Check sheet for the modelled part. Datum: model origin and axes. Units: mm. Face numbers are marked on the shaded views. Coordinates: 2 decimals unless noted, no trailing zeros. Loops run counter-clockwise (first coordinate to the right, second up) from the corner with the lowest first, then second, coordinate; pieces in that order, holes last. Notation, with made-up numbers: (75.25, 12) -> (90.25, 12) arc R20 cw to (90.25, 26) -> close; hole circle Ø4 at (-31, 27). An arc over 180 degrees is marked (long way). Use one line per item in the form item = value.
Autodesk Inventor part; units mm, degrees
ref_plane "YZ Plane" through (0, 0, 0) normal (1, 0, 0) x (0, 1, 0)
ref_plane "XZ Plane" through (0, 0, 0) normal (0, 1, 0) x (-1, 0, 0)
ref_plane "XY Plane" through (0, 0, 0) normal (0, 0, 1) x (1, 0, 0)
sketch "Boceto1" plane through (0, 0, 0) normal (0, 1, 0) x (-1, 0, 0)
  line L0 (-15, 25) -> (15, 25)
  line L1 (15, 25) -> (15, -25)
  line L2 (15, -25) -> (-15, -25)
  line L3 (-15, -25) -> (-15, 25)
  line L4 (-15, 25) -> (15, -25) construction
  line L5 (15, 25) -> (-15, -25) construction
  point P0 (0, 0)
  dimension "d0" = 50
  dimension "d1" = 30
extrude "Extrusión1" add sketch "Boceto1" along normal blind 8
fillet "Empalme1" radius 2 4 edges at (15, 4, 25) (-15, 4, 25) (15, 4, -25) (-15, 4, -25)
sketch "Boceto2" plane through (0, 8, 0) normal (0, 1, 0) x (1, 0, 0)
  circle A0 centre (-9, 19) radius 2.7
  circle A1 centre (9, 19) radius 2.7
  circle A2 centre (9, -19) radius 2.7
  circle A3 centre (-9, -19) radius 2.7
  line L0 (13, 25) -> (-13, 25)
  line L1 (-15, 23) -> (-15, -23)
  line L2 (15, -23) -> (15, 23)
  line L3 (-13, -25) -> (13, -25)
  point P0 (0, 0)
  dimension "d5" = 5.4
  dimension "d6" = 6
  dimension "d7" = 6
  dimension "d8" = 6
  dimension "d9" = 6
extrude "Extrusión2" cut sketch "Boceto2" against normal blind 3
sketch "Boceto3" plane through (0, 0, 0) normal (0, -1, 0) x (1, 0, 0)
  circle A0 centre (0, 19) radius 2.7
  circle A1 centre (0, -19) radius 2.7
  circle A2 centre (-9, -19) radius 2.7
  circle A3 centre (-9, 19) radius 2.7
  point P0 (0, 0)
  dimension "d12" = 5.4
extrude "Extrusión3" cut sketch "Boceto3" against normal through all contours A0 | A1
sketch "Boceto4" plane through (0, 0, 0) normal (0, -1, 0) x (1, 0, 0)
  circle A0 centre (0, -19) radius 2.7
  circle A1 centre (0, -19) radius 4.05
  line L0 (2.3383, -14.95) -> (4.6765, -19)
  line L1 (4.6765, -19) -> (2.3383, -23.05)
  line L2 (2.3383, -23.05) -> (-2.3383, -23.05)
  line L3 (-2.3383, -23.05) -> (-4.6765, -19)
  line L4 (-4.6765, -19) -> (-2.3383, -14.95)
  line L5 (-2.3383, -14.95) -> (2.3383, -14.95)
  circle A2 centre (0, 19) radius 4.05
  line L6 (-4.6765, 19) -> (-2.3383, 23.05)
  line L7 (-2.3383, 23.05) -> (2.3383, 23.05)
  line L8 (2.3383, 23.05) -> (4.6765, 19)
  line L9 (4.6765, 19) -> (2.3383, 14.95)
  line L10 (2.3383, 14.95) -> (-2.3383, 14.95)
  line L11 (-2.3383, 14.95) -> (-4.6765, 19)
  point P0 (0, 0)
  dimension "d15" = 8.1
extrude "Extrusión4" cut sketch "Boceto4" against normal blind 4.5 contours A0 | A1 | A1 L0 L1 | A1 L5 L0 | L1 L2 A1 | A1 L4 L5 | L2 L3 A1 | A1 L3 L4 | A2 | A2 L8 L9 | A2 L7 L8 | L9 L10 A2 | A2 L6 L7 | L10 L11 A2 | A2 L11 L6
properties part number "ViseB"
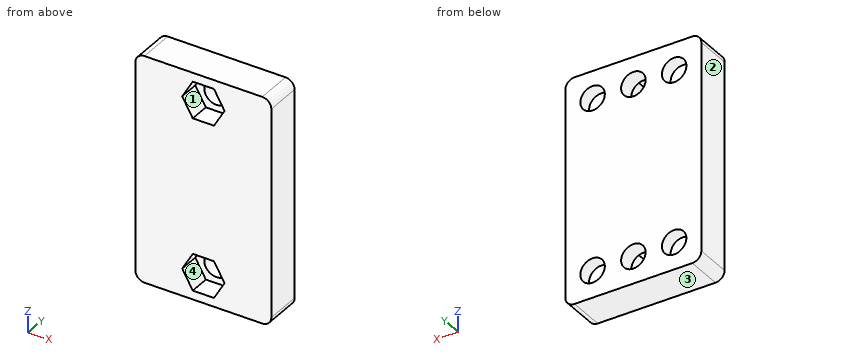
(1) Section check A-A, the plane y = 2.5. Record the boundary of the cut face in (x, z).
Established:
outline = (-15, -23) arc R2 ccw to (-13, -25) -> (13, -25) arc R2 ccw to (15, -23) -> (15, 23) arc R2 ccw to (13, 25) -> (-13, 25) arc R2 ccw to (-15, 23) -> close; hole (-4.68, -19) -> (-2.34, -23.05) -> (2.34, -23.05) -> (4.68, -19) -> (2.34, -14.95) -> (-2.34, -14.95) -> close; hole (-4.68, 19) -> (-2.34, 14.95) -> (2.34, 14.95) -> (4.68, 19) -> (2.34, 23.05) -> (-2.34, 23.05) -> close
(2) Section check D-D, the plane x = 9. Record the boundary of the cut face in (y, z).
Established:
outline = (0, -25) -> (8, -25) -> (8, -21.7) -> (5, -21.7) -> (5, -16.3) -> (8, -16.3) -> (8, 16.3) -> (5, 16.3) -> (5, 21.7) -> (8, 21.7) -> (8, 25) -> (0, 25) -> close
(3) Section check C-C, the plane y = 6. Record the boundary of the cut face in (x, z), plus the area to 3 significant figures.
Established:
outline = (-15, -23) arc R2 ccw to (-13, -25) -> (13, -25) arc R2 ccw to (15, -23) -> (15, 23) arc R2 ccw to (13, 25) -> (-13, 25) arc R2 ccw to (-15, 23) -> close; hole circle Ø5.4 at (-9, -19); hole circle Ø5.4 at (-9, 19); hole circle Ø5.4 at (0, -19); hole circle Ø5.4 at (0, 19); hole circle Ø5.4 at (9, -19); hole circle Ø5.4 at (9, 19)
area = 1,360 mm²
(4) Mould release check, pull along Z, two halves, no side actions. Record for the marked faces 1, 2, 3 and 4: +Z half, -Z half, draft (parallel to the pull), parting line (faces both ways), or undercut.
Established:
face_1 = undercut
face_2 = draft
face_3 = -Z half
face_4 = undercut
(5) Go/stop test with flat-tipped pins: P1, Ø5, axis at x = 0, z = 19, coming from the -Y side; P2, Ø1.6, axis at x = 9.5, z = -18.5, coming from the +Y side. Record where each tip stops, or that it passes through.
Established:
P1 = through
P2 = 5
(6) Section check B-B, the plane z = 18. Record the boundary of the cut face in (x, y).
Established:
outline = (-15, 0) -> (-4.1, 0) -> (-4.1, 4.5) -> (-2.51, 4.5) -> (-2.51, 8) -> (-6.49, 8) -> (-6.49, 5) -> (-11.51, 5) -> (-11.51, 8) -> (-15, 8) -> close; (2.51, 4.5) -> (4.1, 4.5) -> (4.1, 0) -> (15, 0) -> (15, 8) -> (11.51, 8) -> (11.51, 5) -> (6.49, 5) -> (6.49, 8) -> (2.51, 8) -> close
(7) Scan lines: line 1 along Z through (x, y) = (9, 6.6); line 2 along Z through (x, y) = (0, 2.75); line 3 along X through (y, z) = (6.25, 17). Record each from-to range of solid material in increasing order.
Established:
line_1 = -25 to -21.7, -16.3 to 16.3, 21.7 to 25
line_2 = -25 to -23.05, -14.95 to 14.95, 23.05 to 25
line_3 = -15 to -10.81, -7.19 to -1.81, 1.81 to 7.19, 10.81 to 15
